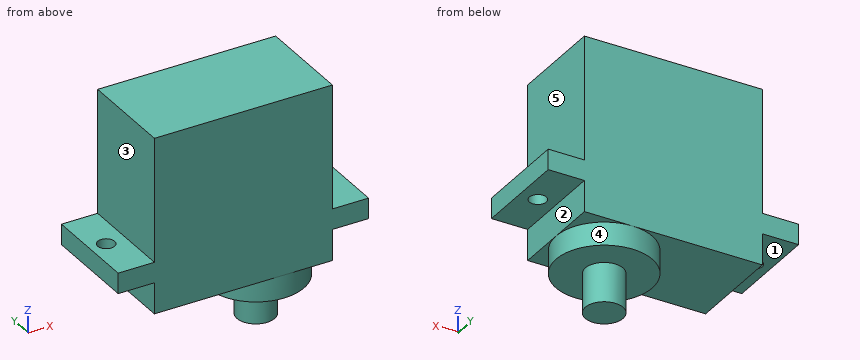
from build123d import *

# Parameters (mm, degrees)
SKETCH_1_R          = 6.25
SKETCH_1_R_2        = 2.45
EXTRUDE_1_DEPTH     = 16.1
SKETCH_1_3_W        = 32.5
SKETCH_1_3_H        = 12.5
EXTRUDE_2_DEPTH     = 2.66
SKETCH_1_4_R        = 6.25
SKETCH_1_4_R_2      = 2.45
SKETCH_1_4_W        = 23.1
SKETCH_1_4_H        = 12.5
EXTRUDE_3_DEPTH     = 6.7
SKETCH_1_5_R        = 6.25
EXTRUDE_4_DEPTH     = 9.7
SKETCH_1_6_R        = 2.45
EXTRUDE_5_DEPTH     = 14.8
SKETCH_3_R          = 1.1
CUT_EXTRUDE_1_DEPTH = 14.8
SKETCH_2_R          = 1.1
CUT_EXTRUDE_2_DEPTH = 14.8


with BuildPart() as part:
    # 草图1 → 凸台-拉伸1 (new body)
    with BuildSketch(Plane.XY):
        with BuildLine():
            Line((4.7, 12.5), (4.7, 0))
            Line((4.7, 0), (21.55, 0))
            ThreePointArc((21.55, 0), (15.3, 6.25), (21.55, 12.5))
            Line((21.55, 12.5), (4.7, 12.5))
        make_face()
        with BuildLine():
            Line((27.8, 12.5), (21.55, 12.5))
            ThreePointArc((21.55, 12.5), (25.969417382, 10.669417382), (27.8, 6.25))
            Line((27.8, 6.25), (27.8, 12.5))
        make_face()
        with BuildLine():
            ThreePointArc((27.8, 6.25), (25.969417382, 1.830582618), (21.55, 0))
            Line((21.55, 0), (27.8, 0))
            Line((27.8, 0), (27.8, 6.25))
        make_face()
        with Locations((21.55, 6.25)):
            Circle(SKETCH_1_R)
        with Locations((21.55, 6.25)):
            Circle(SKETCH_1_R_2, mode=Mode.SUBTRACT)
        with Locations((21.55, 6.25)):
            Circle(SKETCH_1_R_2)
    extrude(amount=EXTRUDE_1_DEPTH)

    # 草图1<3> → 凸台-拉伸2 (add)
    with BuildSketch(Plane.XY):
        with Locations((16.25, 6.25)):
            Rectangle(SKETCH_1_3_W, SKETCH_1_3_H)
    extrude(amount=-EXTRUDE_2_DEPTH)

    # 草图1<4> → 凸台-拉伸3 (add)
    with BuildSketch(Plane.XY):
        with Locations((21.55, 6.25)):
            Circle(SKETCH_1_4_R)
        with Locations((21.55, 6.25)):
            Circle(SKETCH_1_4_R_2, mode=Mode.SUBTRACT)
        with Locations((16.25, 6.25)):
            Rectangle(SKETCH_1_4_W, SKETCH_1_4_H)
    extrude(amount=-EXTRUDE_3_DEPTH)

    # 草图1<5> → 凸台-拉伸4 (add)
    with BuildSketch(Plane.XY):
        with Locations((21.55, 6.25)):
            Circle(SKETCH_1_5_R)
    extrude(amount=-EXTRUDE_4_DEPTH)

    # 草图1<6> → 凸台-拉伸5 (add)
    with BuildSketch(Plane.XY):
        with Locations((21.55, 6.25)):
            Circle(SKETCH_1_6_R)
    extrude(amount=-EXTRUDE_5_DEPTH)

    # 草图3 → 切除-拉伸1 (cut)
    with BuildSketch(Plane(origin=(0, 0, -2.66), x_dir=(-1, 0, 0), z_dir=(0, 0, -1))):
        with Locations((-2.12941164, 6.25)):
            Circle(SKETCH_3_R)
    extrude(amount=-CUT_EXTRUDE_1_DEPTH, mode=Mode.SUBTRACT)

    # 草图2 → 切除-拉伸2 (cut)
    with BuildSketch(Plane(origin=(0, 0, -2.66), x_dir=(-1, 0, 0), z_dir=(0, 0, -1))):
        with Locations((-30.15, 6.25)):
            Circle(SKETCH_2_R)
    extrude(amount=-CUT_EXTRUDE_2_DEPTH, mode=Mode.SUBTRACT)


solid = part.part
Verification items for the finished model (mm, model axes). Face numbers are marked on the shaded views. A direction names the side the tool comes from. Coordinates: 2 decimals unless noted, no trailing zeros. Loops run counter-clockwise (first coordinate to the right, second up) from the corner with the lowest first, then second, coordinate; pieces in that order, holes last. Notation, with made-up numbers: (-4, 21.5) -> (32, 21.5) arc R12 cw to (32, 43.5) -> close; hole circle Ø3 at (-13.75, -37.5). An arc over 180 degrees is marked (long way). Write each question's results on one line, items separated by ' | '.
Item 1: Gauge pin test, flat ends, axial feed: pin 1 (2.5 mm diameter, centred on x = 3, y = 5.5, fed in from -Z); pin 2 (2.5 mm diameter, centred on x = 31, y = 7, fed in from +Z); pin 3 (6 mm diameter, centred on y = 4.5, z = 5.5, fed in from -X). Record the tip position at first contact, or that the pin passes through.
Found:
pin 1: stops at z = -2.66 | pin 2: stops at z = 0 | pin 3: stops at x = 4.7
Item 2: Section check A-A, the plane x = 30.15. Enter the section's corners in (y, z), plus the area to 3 significant figures.
Found:
outline: (0, -2.66) -> (5.15, -2.66) -> (5.15, 0) -> (0, 0) -> close; (7.35, -2.66) -> (12.5, -2.66) -> (12.5, 0) -> (7.35, 0) -> close | area: 27.4 mm2
Item 3: Section check D-D, the plane y = 8. Enter the section's corners in (x, z), plus the area to 3 significant figures.
Found:
outline: (0, -2.66) -> (4.7, -2.66) -> (4.7, -6.7) -> (15.55, -6.7) -> (15.55, -9.7) -> (19.84, -9.7) -> (19.84, -14.8) -> (23.26, -14.8) -> (23.26, -9.7) -> (27.55, -9.7) -> (27.55, -6.7) -> (27.8, -6.7) -> (27.8, -2.66) -> (32.5, -2.66) -> (32.5, 0) -> (27.8, 0) -> (27.8, 16.1) -> (4.7, 16.1) -> (4.7, 0) -> (0, 0) -> close | area: 605 mm2
Item 4: Tool access check on the marked faces 1, 2, 3, 4 and 5. Record the directions out of +Z, -Z, +X, -X, +Y, -Y that give a thin tool (end or side, any length) a straight path to the whole face; none if there is none.
Found:
face 1: -Z, -X, +Y, -Y | face 2: -Z, +X, +Y, -Y | face 3: +Z, -X, +Y, -Y | face 4: -Z | face 5: +Z, +X, +Y, -Y
Item 5: Material ranges on L1, parallel to Y at x = 30.15, z = -1.3; L2, parallel to Z at x = 26.5, y = 8.5; L3, parallel to Z at x = 31, y = 7, recorded low to high.
Found:
L1: y = 0 to 5.15, 7.35 to 12.5 | L2: z = -9.7 to 16.1 | L3: z = -2.66 to 0
Item 6: Section check B-B, the plane y = 3. Enter the section's corners in (x, z).
Found:
outline: (0, -2.66) -> (4.7, -2.66) -> (4.7, -6.7) -> (16.21, -6.7) -> (16.21, -9.7) -> (26.89, -9.7) -> (26.89, -6.7) -> (27.8, -6.7) -> (27.8, -2.66) -> (32.5, -2.66) -> (32.5, 0) -> (27.8, 0) -> (27.8, 16.1) -> (4.7, 16.1) -> (4.7, 0) -> (0, 0) -> close
Item 7: Section check C-C, the plane z = -5. Enter the section's corners in (x, y), plus the area to 3 significant figures.
Found:
outline: (4.7, 0) -> (27.8, 0) -> (27.8, 12.5) -> (4.7, 12.5) -> close | area: 289 mm2
